Geometry check sheet. Reference: the model listing, model coordinates, mm. A direction names the side the tool comes from. Give positions to 0.01 mm unless a question says otherwise; leave off trailing zeros. Write each loop counter-clockwise with the first axis right and the second up, starting at its lowest first coordinate (ties: lowest second). Pieces come first, ordered by that corner, then holes. Notation, with made-up numbers: (25.5, 49) - (66.5, 49) arc R9 cw to (66.5, 64) - close; hole circle Ø8 at (3.25, -10). An arc over 180 degrees is marked (long way). One line per question, with ' | ' between items. Start each with the question number.
Q1. Set-up check for faces 5 (the face through (-76, 2, -49.5)), 6 (the face through (-74, -125.5, 1)), 7 (the face through (-74, 147, 47.5)), 8 (the face through (-74, 123.5, 1)): record each of +Z, -Z, +X, -X, +Y, -Y from which the full face is reachable in a straight line by a thin tool's end or side.
Q2. Section check A-A on z = 35. Record the boundary of the cut face in (x, y), and give its area (3 significant figures).
Q3. Thickness scan on L1, parallel to Y at x = -129, z = 17.5; L2, parallel to Z at x = -33.5, y = -10; L3, parallel to Y at x = -32.7, z = -48.4 (3 decimals). Record the ranges inside material, lowest first. Write a range as [from, to].
Q4. Section check C-C on x = -109.5. Record the boundary of the cut face in (y, z), and give its area (3 significant figures).
Q5. Section check D-D on y = -17.5. Record the boundary of the cut face in (x, z), and give its area (3 significant figures).
Q6. Section check B-B on z = -14. Record the boundary of the cut face in (x, y), and give its area (3 significant figures).
Q7. Release check for a two-part mould opening along Z. For faces 1 (the face through (-76, 148, 49.5)), 2 (the face through (-74, -148, 47.5)), 3 (the face through (-64.576, -124.486, -7.993)), 4 (the face through (-74, -123.5, 1)) record: +Z half, -Z half, draft (parallel to the pull), parting line (faces both ways), or undercut.
Q8. Gauge pin test, flat ends, axial feed: P1, Ø10, axis at y = -52, z = -39.5, coming from the -X side; P2, Ø4.5, axis at x = -117.3, y = -72.9, coming from the +Z side; P3, Ø8, axis at x = -66, z = 29, coming from the -Y side; P4, Ø12, axis at x = -94.5, y = 138, coming from the -Z side. Record the tip position at first contact, or that the pin passes through.
```python
from build123d import *

# Parameters (mm, degrees)
SKETCH_1_W           = 123
SKETCH_1_H           = 335
EXTRUDE_1_DEPTH      = 99
SKETCH_2_W           = 97
SKETCH_2_H           = 247
CUT_EXTRUDE_1_DEPTH  = 214.62467086
SKETCH_3_W           = 97
SKETCH_3_H           = 42
CUT_EXTRUDE_2_DEPTH  = 214.62467086
SKETCH_4_W           = 97
SKETCH_4_H           = 42
CUT_EXTRUDE_3_DEPTH  = 214.62467086
CUT_EXTRUDE_4_DEPTH  = 238.675198538
CUT_EXTRUDE_5_DEPTH  = 237.849108084
CUT_EXTRUDE_6_DEPTH  = 238.675198538
CUT_EXTRUDE_7_DEPTH  = 237.849108084
HOLE_WIZARD_M4_1_D   = 4
HOLE_WIZARD_M4_2_D   = 4
HOLE_WIZARD_M4_3_D   = 4
HOLE_WIZARD_M4_4_D   = 4
HOLE_WIZARD_M4_5_D   = 4
HOLE_WIZARD_M4_6_D   = 4
HOLE_WIZARD_M4_7_D   = 4
HOLE_WIZARD_M4_8_D   = 4
HOLE_WIZARD_9_D      = 40
HOLE_WIZARD_9_DEPTH  = 2
HOLE_WIZARD_10_D     = 40
HOLE_WIZARD_10_DEPTH = 2
HOLE_WIZARD_11_D     = 40
HOLE_WIZARD_11_DEPTH = 293
HOLE_WIZARD_12_D     = 40
HOLE_WIZARD_12_DEPTH = 293
FILLET_1_R           = 2
FILLET_2_R           = 2
FILLET_3_R           = 2
FILLET_4_R           = 2
FILLET_5_R           = 4
FILLET_6_R           = 4
FILLET_7_R           = 4
FILLET_8_R           = 4
FILLET_9_R           = 5
FILLET_10_R          = 5
FILLET_11_R          = 5
FILLET_12_R          = 5


with BuildPart() as part:
    # 草图1 → 凸台-拉伸1 (new body)
    with BuildSketch(Plane.XY.offset(49.5)):
        with Locations((-75, 0)):
            Rectangle(SKETCH_1_W, SKETCH_1_H)
    extrude(amount=-EXTRUDE_1_DEPTH)

    # 草图2 → 切除-拉伸1 (cut, through all)
    with BuildSketch(Plane(origin=(-13.5, 0, 0), x_dir=(0, 0, -1), z_dir=(1, 0, 0))):
        with Locations((-1, 0)):
            Rectangle(SKETCH_2_W, SKETCH_2_H)
    extrude(amount=-CUT_EXTRUDE_1_DEPTH, mode=Mode.SUBTRACT)

    # 草图3 → 切除-拉伸2 (cut, through all)
    with BuildSketch(Plane(origin=(-13.5, 0, 0), x_dir=(0, 0, -1), z_dir=(1, 0, 0))):
        with Locations((1, 146.5)):
            Rectangle(SKETCH_3_W, SKETCH_3_H)
    extrude(amount=-CUT_EXTRUDE_2_DEPTH, mode=Mode.SUBTRACT)

    # 草图4 → 切除-拉伸3 (cut, through all)
    with BuildSketch(Plane(origin=(-13.5, 0, 0), x_dir=(0, 0, -1), z_dir=(1, 0, 0))):
        with Locations((1, -146.5)):
            Rectangle(SKETCH_4_W, SKETCH_4_H)
    extrude(amount=-CUT_EXTRUDE_3_DEPTH, mode=Mode.SUBTRACT)

    # 草图5 → 切除-拉伸4 (cut, through all)
    with BuildSketch(Plane.XY.offset(49.5)):
        with BuildLine():
            Line((-30.75, 142.5), (-30.75, 152.5))
            ThreePointArc((-30.75, 152.5), (-33.5, 155.25), (-36.25, 152.5))
            Line((-36.25, 152.5), (-36.25, 142.5))
            ThreePointArc((-36.25, 142.5), (-33.5, 139.75), (-30.75, 142.5))
        make_face()
    extrude(amount=-CUT_EXTRUDE_4_DEPTH, mode=Mode.SUBTRACT)

    # 草图6 → 切除-拉伸5 (cut, through all)
    with BuildSketch(Plane(origin=(0, 0, 47.5), x_dir=(-1, 0, 0), z_dir=(0, 0, -1))):
        with BuildLine():
            Line((113.75, 152.5), (113.75, 142.5))
            ThreePointArc((113.75, 142.5), (116.5, 139.75), (119.25, 142.5))
            Line((119.25, 142.5), (119.25, 152.5))
            ThreePointArc((119.25, 152.5), (116.5, 155.25), (113.75, 152.5))
        make_face()
    extrude(amount=-CUT_EXTRUDE_5_DEPTH, mode=Mode.SUBTRACT)

    # 草图7 → 切除-拉伸6 (cut, through all)
    with BuildSketch(Plane.XY.offset(49.5)):
        with BuildLine():
            Line((-30.75, -152.5), (-30.75, -142.5))
            ThreePointArc((-30.75, -142.5), (-33.5, -139.75), (-36.25, -142.5))
            Line((-36.25, -142.5), (-36.25, -152.5))
            ThreePointArc((-36.25, -152.5), (-33.5, -155.25), (-30.75, -152.5))
        make_face()
    extrude(amount=-CUT_EXTRUDE_6_DEPTH, mode=Mode.SUBTRACT)

    # 草图8 → 切除-拉伸7 (cut, through all)
    with BuildSketch(Plane(origin=(0, 0, 47.5), x_dir=(-1, 0, 0), z_dir=(0, 0, -1))):
        with BuildLine():
            Line((113.75, -142.5), (113.75, -152.5))
            ThreePointArc((113.75, -152.5), (116.5, -155.25), (119.25, -152.5))
            Line((119.25, -152.5), (119.25, -142.5))
            ThreePointArc((119.25, -142.5), (116.5, -139.75), (113.75, -142.5))
        make_face()
    extrude(amount=-CUT_EXTRUDE_7_DEPTH, mode=Mode.SUBTRACT)

    # M4 螺纹孔1 (through all)
    with Locations(Plane.XY.offset(-47.5)):
        with Locations((-117.3, -72.9)):
            Hole(HOLE_WIZARD_M4_1_D / 2)

    # M4 螺纹孔2 (through all)
    with Locations(Plane.XY.offset(-47.5)):
        with Locations((-91.7, -72.9)):
            Hole(HOLE_WIZARD_M4_2_D / 2)

    # M4 螺纹孔3 (through all)
    with Locations(Plane.XY.offset(-47.5)):
        with Locations((-32.7, -72.9)):
            Hole(HOLE_WIZARD_M4_3_D / 2)

    # M4 螺纹孔4 (through all)
    with Locations(Plane.XY.offset(-47.5)):
        with Locations((-58.3, -72.9)):
            Hole(HOLE_WIZARD_M4_4_D / 2)

    # M4 螺纹孔5 (through all)
    with Locations(Plane.XY.offset(-47.5)):
        with Locations((-91.7, 102.9)):
            Hole(HOLE_WIZARD_M4_5_D / 2)

    # M4 螺纹孔6 (through all)
    with Locations(Plane.XY.offset(-47.5)):
        with Locations((-117.3, 102.9)):
            Hole(HOLE_WIZARD_M4_6_D / 2)

    # M4 螺纹孔7 (through all)
    with Locations(Plane.XY.offset(-47.5)):
        with Locations((-32.7, 102.9)):
            Hole(HOLE_WIZARD_M4_7_D / 2)

    # M4 螺纹孔8 (through all)
    with Locations(Plane.XY.offset(-47.5)):
        with Locations((-58.3, 102.9)):
            Hole(HOLE_WIZARD_M4_8_D / 2)

    # 孔9
    with Locations(Plane.XZ.offset(125.5)):
        with Locations((-45.5, -14)):
            Hole(HOLE_WIZARD_9_D / 2, depth=HOLE_WIZARD_9_DEPTH)

    # 孔10
    with Locations(Plane.XZ.offset(125.5)):
        with Locations((-104.5, -14)):
            Hole(HOLE_WIZARD_10_D / 2, depth=HOLE_WIZARD_10_DEPTH)

    # 孔11
    with Locations(Plane(origin=(0, 125.5, 0), x_dir=(-1, 0, 0), z_dir=(0, 1, 0))):
        with Locations((104.5, -14)):
            Hole(HOLE_WIZARD_11_D / 2, depth=HOLE_WIZARD_11_DEPTH)

    # 孔12
    with Locations(Plane(origin=(0, 125.5, 0), x_dir=(-1, 0, 0), z_dir=(0, 1, 0))):
        with Locations((45.5, -14)):
            Hole(HOLE_WIZARD_12_D / 2, depth=HOLE_WIZARD_12_DEPTH)

    # 圆角1
    fillet_1_edges = [part.edges().sort_by_distance(p)[0] for p in [
        (-75, 125.5, 47.5),
    ]]
    fillet(fillet_1_edges, radius=FILLET_1_R)

    # 圆角2
    fillet_2_edges = [part.edges().sort_by_distance(p)[0] for p in [
        (-75, -125.5, 47.5),
    ]]
    fillet(fillet_2_edges, radius=FILLET_2_R)

    # 圆角3
    fillet_3_edges = [part.edges().sort_by_distance(p)[0] for p in [
        (-75, -123.5, -47.5),
    ]]
    fillet(fillet_3_edges, radius=FILLET_3_R)

    # 圆角4
    fillet_4_edges = [part.edges().sort_by_distance(p)[0] for p in [
        (-75, 123.5, -47.5),
    ]]
    fillet(fillet_4_edges, radius=FILLET_4_R)

    # 圆角5
    fillet_5_edges = [part.edges().sort_by_distance(p)[0] for p in [
        (-75, 123.5, 49.5),
    ]]
    fillet(fillet_5_edges, radius=FILLET_5_R)

    # 圆角6
    fillet_6_edges = [part.edges().sort_by_distance(p)[0] for p in [
        (-75, -123.5, 49.5),
    ]]
    fillet(fillet_6_edges, radius=FILLET_6_R)

    # 圆角7
    fillet_7_edges = [part.edges().sort_by_distance(p)[0] for p in [
        (-75, -125.5, -49.5),
    ]]
    fillet(fillet_7_edges, radius=FILLET_7_R)

    # 圆角8
    fillet_8_edges = [part.edges().sort_by_distance(p)[0] for p in [
        (-75, 125.5, -49.5),
    ]]
    fillet(fillet_8_edges, radius=FILLET_8_R)

    # 圆角9
    fillet_9_edges = [part.edges().sort_by_distance(p)[0] for p in [
        (-136.5, -167.5, 48.5),
    ]]
    fillet(fillet_9_edges, radius=FILLET_9_R)

    # 圆角10
    fillet_10_edges = [part.edges().sort_by_distance(p)[0] for p in [
        (-136.5, 167.5, 48.5),
    ]]
    fillet(fillet_10_edges, radius=FILLET_10_R)

    # 圆角11
    fillet_11_edges = [part.edges().sort_by_distance(p)[0] for p in [
        (-13.5, -167.5, 48.5),
    ]]
    fillet(fillet_11_edges, radius=FILLET_11_R)

    # 圆角12
    fillet_12_edges = [part.edges().sort_by_distance(p)[0] for p in [
        (-13.5, 167.5, 48.5),
    ]]
    fillet(fillet_12_edges, radius=FILLET_12_R)


solid = part.part
```
Working result:
1) face 5: -Z, +X, -X, +Y, -Y | face 6: -Z, +X, -X, -Y | face 7: -Z, +X, -X, +Y | face 8: +Z, +X, -X
2) outline: (-136.5, -125.5) - (-13.5, -125.5) - (-13.5, -123.5) - (-136.5, -123.5) - close; (-136.5, 123.5) - (-13.5, 123.5) - (-13.5, 125.5) - (-136.5, 125.5) - close | area: 492 mm2
3) L1: y = [-125.5, -123.5], [123.5, 125.5] | L2: z = [-49.5, -47.5] | L3: y = [-124.255, -74.9], [-70.9, 100.9], [104.9, 124.255]
4) outline: (-167.5, 47.5) - (-127.5, 47.5) arc R2 cw to (-125.5, 45.5) - (-125.5, 5.36) - (-123.5, 5.36) - (-123.5, 45.5) arc R4 ccw to (-127.5, 49.5) - (-167.5, 49.5) - close; (-125.5, -45.5) arc R4 ccw to (-121.5, -49.5) - (121.5, -49.5) arc R4 ccw to (125.5, -45.5) - (125.5, -33.36) - (123.5, -33.36) - (123.5, -45.5) arc R2 cw to (121.5, -47.5) - (-121.5, -47.5) arc R2 cw to (-123.5, -45.5) - (-123.5, -33.36) - (-125.5, -33.36) - close; (123.5, 5.36) - (125.5, 5.36) - (125.5, 45.5) arc R2 cw to (127.5, 47.5) - (167.5, 47.5) - (167.5, 49.5) - (127.5, 49.5) arc R4 ccw to (123.5, 45.5) - close | area: 893 mm2
5) outline: (-136.5, -49.5) - (-13.5, -49.5) - (-13.5, -47.5) - (-136.5, -47.5) - close | area: 246 mm2
6) outline: (-136.5, -125.5) - (-124.5, -125.5) - (-124.5, -123.5) - (-136.5, -123.5) - close; (-136.5, 123.5) - (-124.5, 123.5) - (-124.5, 125.5) - (-136.5, 125.5) - close; (-84.5, -125.5) - (-65.5, -125.5) - (-65.5, -123.5) - (-84.5, -123.5) - close; (-84.5, 123.5) - (-65.5, 123.5) - (-65.5, 125.5) - (-84.5, 125.5) - close; (-25.5, -125.5) - (-13.5, -125.5) - (-13.5, -123.5) - (-25.5, -123.5) - close; (-25.5, 123.5) - (-13.5, 123.5) - (-13.5, 125.5) - (-25.5, 125.5) - close | area: 172 mm2
7) face 1: +Z half | face 2: -Z half | face 3: undercut | face 4: draft
8) P1: passes through | P2: stops at z = -47.5 | P3: stops at y = -125.5 | P4: stops at z = 47.5
